Here's the drawing with two shaded views (mm, measured from the low corner). I have some questions. Round coordinates to 2 decimals unless told otherwise and drop trailing zeros. Order: outer loops, then holes, each group sorted by start corner. A loop starts at its lowest first (then second) coordinate and runs counter-clockwise, first axis right, second up. Notation, with made-up numbers: (68.5, 70.5) - (91.5, 70.5) arc R24 ccw to (91.5, 83.5) - close; hole circle Ø4 at (4, 89). An arc over 180 degrees is marked (long way). Return JSON: item names as keys, results as strings. Group by question number.
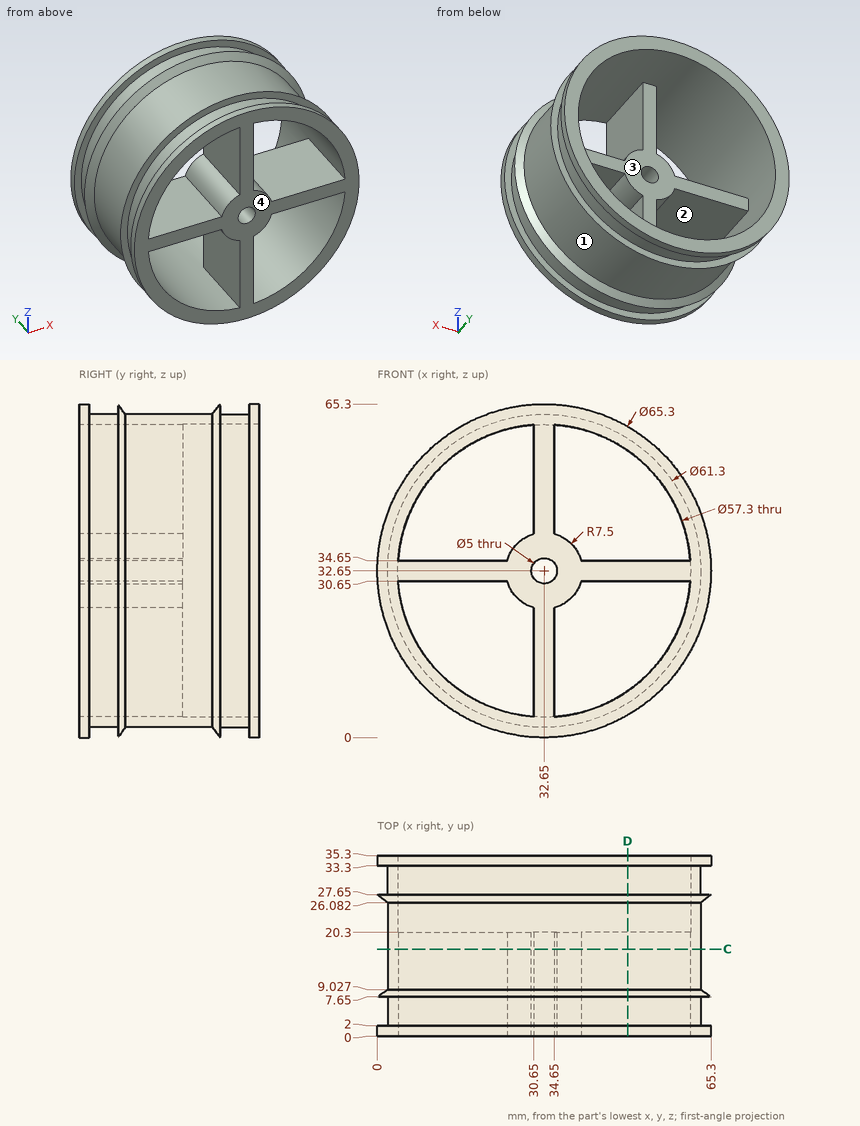
1) We'd pull the mould along Y, two halves only. Please class the marked faces 1, 2, 3 and 4: +Y half, -Y half, draft (parallel to the pull), parting line (faces both ways), or undercut.
2) I want a section at C-C, the plane y = 17. List the corners of the cut face in (x, z) for me.
3) Will these pins go through, and if not, where does the flat tip stop? pin 1 (8 mm diameter, centred on x = 32.65, z = 32.65, fed in from +Y); pin 2 (10 mm diameter, centred on y = 10, z = 51.5, fed in from -X) (1 decimal); pin 3 (6 mm diameter, centred on x = 54.5, y = 8, fed in from +Z) (1 decimal); pin 4 (3 mm diameter, centred on x = 27, z = 41.5, fed in from +Y).
4) I want a section at D-D, the plane x = 49. Give the number of separate pieces and of enclosed holes in the cut face, plus the area to 3 significant figures.
5) If I drill on line 1 along Z through (x, y) = (32.65, 21.5); line 2 along X through (y, z) = (13.25, 32.65); line 3 along X through (y, z) = (26, 32), over which ranges is the centre line in solid material (lowest first)? Write a range as from..to.
Outcome:
{
 "1": {"face 1": "undercut", "face 2": "draft", "face 3": "+Y half", "face 4": "-Y half"},
 "2": {"outline": "circle Ø61.3 at (32.65, 32.65); hole (4.07, 30.65) arc R28.65 ccw to (30.65, 4.07) - (30.65, 25.42) arc R7.5 cw to (25.42, 30.65) - close; hole (4.07, 34.65) - (25.42, 34.65) arc R7.5 cw to (30.65, 39.88) - (30.65, 61.23) arc R28.65 ccw to start; hole circle Ø5 at (32.65, 32.65); hole (34.65, 4.07) arc R28.65 ccw to (61.23, 30.65) - (39.88, 30.65) arc R7.5 cw to (34.65, 25.42) - close; hole (34.65, 39.88) arc R7.5 cw to (39.88, 34.65) - (61.23, 34.65) arc R28.65 ccw to (34.65, 61.23) - close"},
 "3": {"pin 1": "y = 20.3", "pin 2": "x = 3.4", "pin 3": "z = 59.3", "pin 4": "through"},
 "4": {"separate pieces": "3", "enclosed holes": "0", "area": "276 mm^2"},
 "5": {"line 1": "2..4, 61.3..63.3", "line 2": "2..30.15, 35.15..63.3", "line 3": "2.01..4.01, 61.29..63.29"}
}
